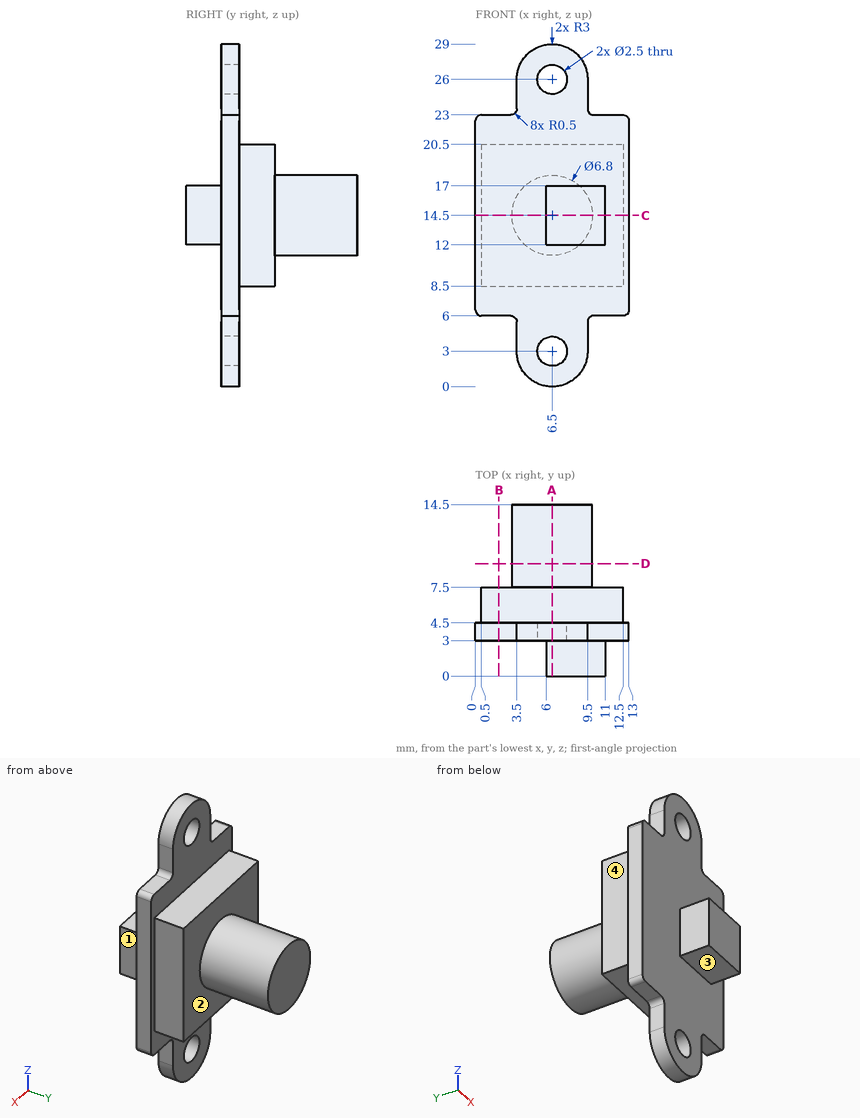
The figure shows three views and two pictorial views of one solid part (mm, origin at its lowest corner). Answer the questions. A direction names the side the tool comes from. Coordinates: 2 decimals unless noted, no trailing zeros. Loops run counter-clockwise (first coordinate to the right, second up) from the corner with the lowest first, then second, coordinate; pieces in that order, holes last. Notation, with made-up numbers: (67.5, 32) -> (98.5, 32) arc R14 ccw to (98.5, 59) -> close; hole circle Ø11 at (-12.5, 9). An arc over 180 degrees is marked (long way). Write item = value, one per line. Start each with the question number.
1) Given pin 1 Ø0.9 at (x, y) = (9.5, 1.5) entering from +Z; pin 2 Ø6 at (x, y) = (10, 12.5) entering from -Z; pin 3 Ø1.6 at (y, z) = (3.5, 5) entering from +X, each flat-ended and moving along its own axis, determine where each tip first touches the part or whether it passes through.
2) A cutting plane is placed at C-C (z = 14.5). Give the vertices of the cut face in (x, y), then the cut area to 3 significant figures.
3) A cutting plane is placed at A-A (x = 6.5). Give the vertices of the cut face in (y, z).
4) Straight lines are drawn through the part: line 1 (X direction, y = 4.15, z = 26); line 2 (Z direction, x = 6.5, y = 3.45); line 3 (Z direction, x = 7.25, y = 3.5). For each, find the intervals that lie inside material, in ascending order. Write a range as from..to.
5) A cutting plane is placed at B-B (x = 2). Give the vertices of the cut face in (y, z), then the cut area to 3 significant figures.
6) A tool of negligible diameter and unlimited length cuts with its end or side. For the marked faces 1, 2, 3 and 4, from which of +Z, -Z, +X, -X, +Y, -Y can it reach the whole face along a straight path? Write none if from no direction.
7) A cutting plane is placed at D-D (y = 9.5). Give the vertices of the cut face in (x, z), then the cut area to 3 significant figures.
Responses:
q1.pin_1 = 17
q1.pin_2 = 11.14
q1.pin_3 = 9.6
q2.outline = (0, 3) -> (6, 3) -> (6, 0) -> (11, 0) -> (11, 3) -> (13, 3) -> (13, 4.5) -> (12.5, 4.5) -> (12.5, 7.5) -> (9.9, 7.5) -> (9.9, 14.5) -> (3.1, 14.5) -> (3.1, 7.5) -> (0.5, 7.5) -> (0.5, 4.5) -> (0, 4.5) -> close
q2.area = 118 mm²
q3.outline = (0, 12) -> (3, 12) -> (3, 4.25) -> (4.5, 4.25) -> (4.5, 8.5) -> (7.5, 8.5) -> (7.5, 11.1) -> (14.5, 11.1) -> (14.5, 17.9) -> (7.5, 17.9) -> (7.5, 20.5) -> (4.5, 20.5) -> (4.5, 24.75) -> (3, 24.75) -> (3, 17) -> (0, 17) -> close; (3, 0) -> (4.5, 0) -> (4.5, 1.75) -> (3, 1.75) -> close; (3, 27.25) -> (4.5, 27.25) -> (4.5, 29) -> (3, 29) -> close
q4.line_1 = 3.5..5.25, 7.75..9.5
q4.line_2 = 0..1.75, 4.25..24.75, 27.25..29
q4.line_3 = 0.1..2, 4..25, 27..28.9
q5.outline = (3, 6) -> (4.5, 6) -> (4.5, 8.5) -> (7.5, 8.5) -> (7.5, 20.5) -> (4.5, 20.5) -> (4.5, 23) -> (3, 23) -> close
q5.area = 61.5 mm²
q6.face_1 = +Z, -Z, +X, -Y
q6.face_2 = +Y
q6.face_3 = -Z, +X, -X, -Y
q6.face_4 = +Z, -Z, -X, +Y
q7.outline = circle Ø6.8 at (6.5, 14.5)
q7.area = 36.3 mm²
